CAD build for the part. Positions are in the model's coordinates, mm. A direction names the side the tool comes from. Round coordinates to 2 decimals unless told otherwise and drop trailing zeros. Order: outer loops, then holes, each group sorted by start corner. A loop starts at its lowest first (then second) coordinate and runs counter-clockwise, first axis right, second up.
```python
from build123d import *

# Parameters (mm, degrees)
BOSS_EXTRUDE1_DEPTH = 4
SKETCH2_R           = 1
BOSS_EXTRUDE2_DEPTH = 5
CUT_EXTRUDE1_START  = -5
SKETCH2_3_R         = 4
SKETCH2_3_R_2       = 2
SKETCH2_3_R_3       = 1
CUT_EXTRUDE1_DEPTH  = 5
SKETCH3_W           = 22
SKETCH3_H           = 5
BOSS_EXTRUDE3_DEPTH = 17
FILLET1_RADIUS      = 11
FILLET1_LENGTH      = 5
SKETCH5_R           = 2.5
SKETCH5_R_2         = 1.5
CUT_EXTRUDE3_DEPTH  = 17


with BuildPart() as part:
    # Sketch1 → Boss-Extrude1 (new body)
    with BuildSketch(Plane.XY):
        with BuildLine():
            Line((-12.5, 18), (12.5, 18))
            ThreePointArc((12.5, 18), (30.5, 0), (12.5, -18))
            Line((12.5, -18), (-12.5, -18))
            ThreePointArc((-12.5, -18), (-30.5, 0), (-12.5, 18))
        make_face()
    extrude(amount=BOSS_EXTRUDE1_DEPTH)

    # Sketch2 → Boss-Extrude2 (add)
    # profile 1 of 2: a face of its own
    with BuildSketch(Plane.XY.offset(4)):
        with BuildLine():
            Line((-24.5, 6), (-24.5, -6))
            ThreePointArc((-24.5, -6), (-22, -8.5), (-19.5, -6))
            Line((-19.5, -6), (-19.5, 6))
            ThreePointArc((-19.5, 6), (-22, 8.5), (-24.5, 6))
        make_face()
        with Locations((-22, 0)):
            Circle(SKETCH2_R, mode=Mode.SUBTRACT)
    # profile 2 of 2: a face of its own
    with BuildSketch(Plane.XY.offset(4)):
        with BuildLine():
            Line((3.5, 6), (3.5, -6))
            ThreePointArc((3.5, -6), (6, -8.5), (8.5, -6))
            Line((8.5, -6), (8.5, 6))
            ThreePointArc((8.5, 6), (6, 8.5), (3.5, 6))
        make_face()
        with Locations((6, 0)):
            Circle(SKETCH2_R, mode=Mode.SUBTRACT)
    extrude(amount=BOSS_EXTRUDE2_DEPTH)

    # Sketch2<3> → Cut-Extrude1 (cut)
    with BuildSketch(Plane.XY.offset(4).offset(CUT_EXTRUDE1_START)):
        with Locations((-13, 0)):
            Circle(SKETCH2_3_R)
        with Locations((18.110196417, 0)):
            Circle(SKETCH2_3_R_2)
        with Locations((-22, 0)):
            Circle(SKETCH2_3_R_3)
        with Locations((6, 0)):
            Circle(SKETCH2_3_R_3)
    extrude(amount=CUT_EXTRUDE1_DEPTH, mode=Mode.SUBTRACT)

    # Sketch3 → Boss-Extrude3 (add)
    with BuildSketch(Plane.XY.offset(4)):
        with Locations((0, 15.5)):
            Rectangle(SKETCH3_W, SKETCH3_H)
    extrude(amount=BOSS_EXTRUDE3_DEPTH)

    # Fillet1: full round fillet: the end face becomes a half cylinder, R = half its width
    fillet1_face = Plane((0, 15.5, 21), x_dir=(0, 1, 0), z_dir=(0, 0, 1))  # on the end face: x along it, z out of the body
    fillet1_slab = fillet1_face.offset(-FILLET1_RADIUS / 2) * Box(FILLET1_LENGTH, 2 * FILLET1_RADIUS, FILLET1_RADIUS, mode=Mode.PRIVATE)  # the body's end, R deep
    fillet1_round = Plane((0, 15.5, 10), x_dir=(0, 0, 1), z_dir=(0, 1, 0)) * Cylinder(FILLET1_RADIUS, FILLET1_LENGTH, mode=Mode.PRIVATE)  # its axis R under the face
    add(fillet1_slab - fillet1_round, mode=Mode.SUBTRACT)

    # Sketch5 → Cut-Extrude3 (cut)
    with BuildSketch(Plane.XZ.offset(-13)):
        with Locations((0, 11.5)):
            Circle(SKETCH5_R)
        with Locations((5.5, 11.5)):
            Circle(SKETCH5_R_2)
        with Locations((0, 17)):
            Circle(SKETCH5_R_2)
        with Locations((-5.5, 11.5)):
            Circle(SKETCH5_R_2)
        with Locations((0, 6)):
            Circle(SKETCH5_R_2)
    extrude(amount=-CUT_EXTRUDE3_DEPTH, mode=Mode.SUBTRACT)


solid = part.part
```
1. Cut at B-B, the plane x = 0. Write the cut outline in (y, z), and give its area (3 significant figures).
2. Cut at D-D, the plane x = -8. Write the cut outline in (y, z).
3. Pin check, flat tips, straight feed: P1, Ø2.5, axis at x = -22, y = 0, coming from the +Z side; P2, Ø5.5, axis at y = -2.5, z = 6.5, coming from the +X side; P3, Ø4, axis at x = 5.5, z = 11.5, coming from the -Y side. Stop position of each tip, or through.
4. Cut at A-A, the plane z = 6. Write the cut outline in (x, y), and give its area (3 significant figures).
5. Drill centre lines: line 1 (X direction, y = 0, z = 2.25); line 2 (X direction, y = 0, z = 6); line 3 (Y direction, x = 6, z = 4.5). Where is each one in solid material? Low to high.
6. Cut at C-C, the plane z = 11.5. Write the cut outline in (x, y), and give its area (3 significant figures).
7. Mould opens along Y. For faces 1 (the face through (5.9, -8.5, 6.5)), 2 (the face through (6.1, 8.5, 6.5)), 3 (the face through (16.112, 0.088, 1.972)), 4 (the face through (-11, 15, 7)) say: released by +Y, released by -Y, zero draft, split by the parting line, or undercut.
8. Tool access for faces 5 (the face through (-19.5, 0, 6)), 6 (the face through (3.5, 0, 6)), 7 (the face through (4.85, 0.12, 9)), 8 (the face through (11, 15, 7)), 9 (the face through (-21.9, 8.5, 6.5)): list every direction of +Z, -Z, +X, -X, +Y, -Y with a clear straight run to the whole face (end or side of a thin tool).
Outcome:
1. outline: (-18, 0) - (18, 0) - (18, 4.5) - (13, 4.5) - (13, 4) - (-18, 4) - close; (13, 7.5) - (18, 7.5) - (18, 9) - (13, 9) - close; (13, 14) - (18, 14) - (18, 15.5) - (13, 15.5) - close; (13, 18.5) - (18, 18.5) - (18, 21) - (13, 21) - close
1. area: 174 mm2
2. outline: (-18, 0) - (18, 0) - (18, 17.55) - (13, 17.55) - (13, 4) - (-18, 4) - close
3. P1: stops at z = 9
3. P2: stops at x = 30.45
3. P3: stops at y = 13
4. outline: (-24.5, -6) arc R2.5 ccw to (-19.5, -6) - (-19.5, 6) arc R2.5 ccw to (-24.5, 6) - close; (-11, 13) - (-1.5, 13) - (-1.5, 18) - (-11, 18) - close; (1.5, 13) - (11, 13) - (11, 18) - (1.5, 18) - close; (3.5, -6) arc R2.5 ccw to (8.5, -6) - (8.5, 6) arc R2.5 ccw to (3.5, 6) - close; hole circle Ø2 at (-22, 0); hole circle Ø2 at (6, 0)
4. area: 248 mm2
5. line 1: x = -30.5 to -23, -21 to -17, -9 to 5, 7 to 16.11, 20.11 to 30.5
5. line 2: x = -24.5 to -23, -21 to -19.5, 3.5 to 5, 7 to 8.5
5. line 3: y = -8.5 to -1, 1 to 8.5, 13 to 18
6. outline: (-10.9, 13) - (-7, 13) - (-7, 18) - (-10.9, 18) - close; (-4, 13) - (-2.5, 13) - (-2.5, 18) - (-4, 18) - close; (2.5, 13) - (4, 13) - (4, 18) - (2.5, 18) - close; (7, 13) - (10.9, 13) - (10.9, 18) - (7, 18) - close
6. area: 54.0 mm2
7. face 1: released by -Y
7. face 2: undercut
7. face 3: undercut
7. face 4: zero draft
8. face 5: +Z, +Y, -Y
8. face 6: +Z, -Y
8. face 7: +Z, +X, -X, -Y
8. face 8: +Z, +X, +Y, -Y
8. face 9: +Z, +Y
